Geometry check sheet. Reference: the model listing, model coordinates, mm. A direction names the side the tool comes from. Round coordinates to 2 decimals unless told otherwise and drop trailing zeros. Order: outer loops, then holes, each group sorted by start corner. A loop starts at its lowest first (then second) coordinate and runs counter-clockwise, first axis right, second up.
```python
from build123d import *

# Parameters (mm, degrees)
CHANFREIN1_SIZE       = 0.2
EXTRUSION1_DEPTH      = 10
EXTRUSION1_DEPTH_BACK = 10
ESQUISSE2_W           = 4
ESQUISSE2_H           = 1.988568473


with BuildPart() as part:
    # Esquisse1 → R_volution1 (revolve)
    with BuildSketch(Plane.XY, mode=Mode.PRIVATE) as r_volution1_sk:
        Polygon((32, 0), (32, 1.5), (30.8, 1.5), (30.8, 1.15), (30.1, 1.15), (30.1, 1.5), (0, 1.5), (0, 0), align=None)
    revolve(r_volution1_sk.sketch.rotate(Axis((0, 0, 0), (1, 0, 0)), 90), axis=Axis((0, 0, 0), (1, 0, 0)))

    # Chanfrein1
    chanfrein1_edges = [part.edges().sort_by_distance(p)[0] for p in [
        (0, 0, -1.5),
        (32, 0, -1.5),
    ]]
    chamfer(chanfrein1_edges, length=CHANFREIN1_SIZE)

    # Esquisse2 → Extrusion1 (cut, two sides: drawn at the far end of the back side and taken through both)
    with BuildSketch(Plane.XY.offset(-EXTRUSION1_DEPTH_BACK)):
        with Locations((7, 1.994284237)):
            Rectangle(ESQUISSE2_W, ESQUISSE2_H)
    extrude(amount=EXTRUSION1_DEPTH + EXTRUSION1_DEPTH_BACK, mode=Mode.SUBTRACT)


solid = part.part
```
(1) Depth check by flat-ended pin: P1, Ø0.7, axis at x = 7.5, z = -0.5, coming from the +Y side; P2, Ø0.5, axis at y = 1.5, z = 0.5, coming from the +X side. Enter the tip coordinate at first touch or a pass-through.
Returned:
P1: stops at y = 1
P2: stops at x = 31.97
(2) Set-up check for faces 3 (the flat face through (0, 0, 0)), 4 (the cylindrical face through (30.45, 0.7, -0.91)), 5 (the flat face through (7, 1, 0)): record each of +Z, -Z, +X, -X, +Y, -Y from which the full face is reachable in a straight line by a thin tool's end or side.
Returned:
face 3: +Z, -Z, -X, +Y, -Y
face 4: none
face 5: +Z, -Z, +Y
(3) Draft check along Z on faces 1 (the cylindrical face through (31.29, -0.45, 1.43)), 2 (the flat face through (32, 0, 0)). Enter one of: released by +Z, released by -Z, zero draft, split by the parting line, or undercut.
Returned:
face 1: split by the parting line
face 2: zero draft
(4) Material ranges on line 1 (X direction, y = 0.55, z = 1.15); line 2 (Y direction, x = 15.5, z = 0.1); line 3 (Z direction, x = 28, y = 0.75), recorded low to high.
Returned:
line 1: x = 0 to 30.1, 30.8 to 32
line 2: y = -1.5 to 1.5
line 3: z = -1.3 to 1.3
(5) Sectioned sample at B-B, the plane x = 25.5. Record the cut outline in (y, z).
Returned:
outline: circle Ø3 at (0, 0)
(6) Sectioned sample at A-A, the plane z = 0. Record the cut outline in (x, y), and give its area (3 significant figures).
Returned:
outline: (0, -1.3) - (0.2, -1.5) - (30.1, -1.5) - (30.1, -1.15) - (30.8, -1.15) - (30.8, -1.5) - (31.8, -1.5) - (32, -1.3) - (32, 1.3) - (31.8, 1.5) - (30.8, 1.5) - (30.8, 1.15) - (30.1, 1.15) - (30.1, 1.5) - (9, 1.5) - (9, 1) - (5, 1) - (5, 1.5) - (0.2, 1.5) - (0, 1.3) - close
area: 93.4 mm2
